from build123d import *

# Parameters (mm, degrees)
F0_W     = 50
F0_H     = 75
F1_DEPTH = 1200
F2_R     = 5.5
F3_T     = -2.5


with BuildPart() as f1:
    # F0 (on Front) → F1 (new body, symmetric)
    with BuildSketch(Plane.XZ):
        Rectangle(F0_W, F0_H)
    extrude(amount=F1_DEPTH, both=True)

    # F2
    f2_edges = [f1.edges().sort_by_distance(p)[0] for p in [
        (25, 0, 37.5),
        (-25, 0, 37.5),
        (-25, 0, -37.5),
        (25, 0, -37.5),
    ]]
    fillet(f2_edges, radius=F2_R)

    # F3
    f3_openings = [f1.faces().sort_by_distance(p)[0] for p in [
        (0, -1200, 0),
        (0, 1200, 0),
    ]]
    offset(amount=F3_T, openings=f3_openings)


solid = f1.part
Read the model definition and answer for the solid it produces. Units are mm, in the model's axes. A direction names the side the tool comes from. Give positions to 0.01 mm unless a question says otherwise; leave off trailing zeros. Write each loop counter-clockwise with the first axis right and the second up, starting at its lowest first coordinate (ties: lowest second). Pieces come first, ordered by that corner, then holes. Notation, with made-up numbers: (51.25, -30.5) -> (89.25, -30.5) arc R20 ccw to (89.25, -13.5) -> close; hole circle Ø5 at (70.5, 47). An arc over 180 degrees is marked (long way). Answer as a JSON object with one key per item and string values. Group by question number.
1) Find section C-C (x = -6.5). Write down the section's boundary in (y, z).
2) A tool of negligible diameter and unlimited length cuts with its end or side. For faces 1 (the flat face through (-25, -17, 0)), 2 (the flat face through (-22.5, -17, 0)), from which of +Z, -Z, +X, -X, +Y, -Y can it reach the whole face along a straight path? Write none if from no direction.
3) Consider L1, parallel to X at y = -389, z = 31; L2, parallel to Z at x = 0, y = -648; L3, parallel to Z at x = 20.5, y = 1030.5. Determine where each line is inside the solid, lowest interval first. Write a range as from..to.
4) The mould has two halves that part along Z. Classify faces 3 (the flat face through (22.5, -17, 0)), 4 (the flat face through (0, -17, -37.5)), 5 (the flat face through (0, -17, 37.5)): +Z half, -Z half, draft (parallel to the pull), parting line (faces both ways), or undercut.
5) Find section A-A (z = -7.5). Write down the section's boundary in (x, y).
6) Find section B-B (y = 616.5). Write down the section's boundary in (x, z).
Values follow:
{
 "1": {"outline": "(-1200, -37.5) -> (1200, -37.5) -> (1200, -35) -> (-1200, -35) -> close; (-1200, 35) -> (1200, 35) -> (1200, 37.5) -> (-1200, 37.5) -> close"},
 "2": {"face 1": "+Z, -Z, -X, +Y, -Y", "face 2": "+Y, -Y"},
 "3": {"L1": "x = -25..-22.5, 22.5..25", "L2": "z = -37.5..-35, 35..37.5", "L3": "z = -37.41..-34.83, 34.83..37.41"},
 "4": {"face 3": "undercut", "face 4": "-Z half", "face 5": "+Z half"},
 "5": {"outline": "(-25, -1200) -> (-22.5, -1200) -> (-22.5, 1200) -> (-25, 1200) -> close; (22.5, -1200) -> (25, -1200) -> (25, 1200) -> (22.5, 1200) -> close"},
 "6": {"outline": "(-25, -32) arc R5.5 ccw to (-19.5, -37.5) -> (19.5, -37.5) arc R5.5 ccw to (25, -32) -> (25, 32) arc R5.5 ccw to (19.5, 37.5) -> (-19.5, 37.5) arc R5.5 ccw to (-25, 32) -> close; hole (-22.5, -32) arc R3 ccw to (-19.5, -35) -> (19.5, -35) arc R3 ccw to (22.5, -32) -> (22.5, 32) arc R3 ccw to (19.5, 35) -> (-19.5, 35) arc R3 ccw to (-22.5, 32) -> close"}
}
